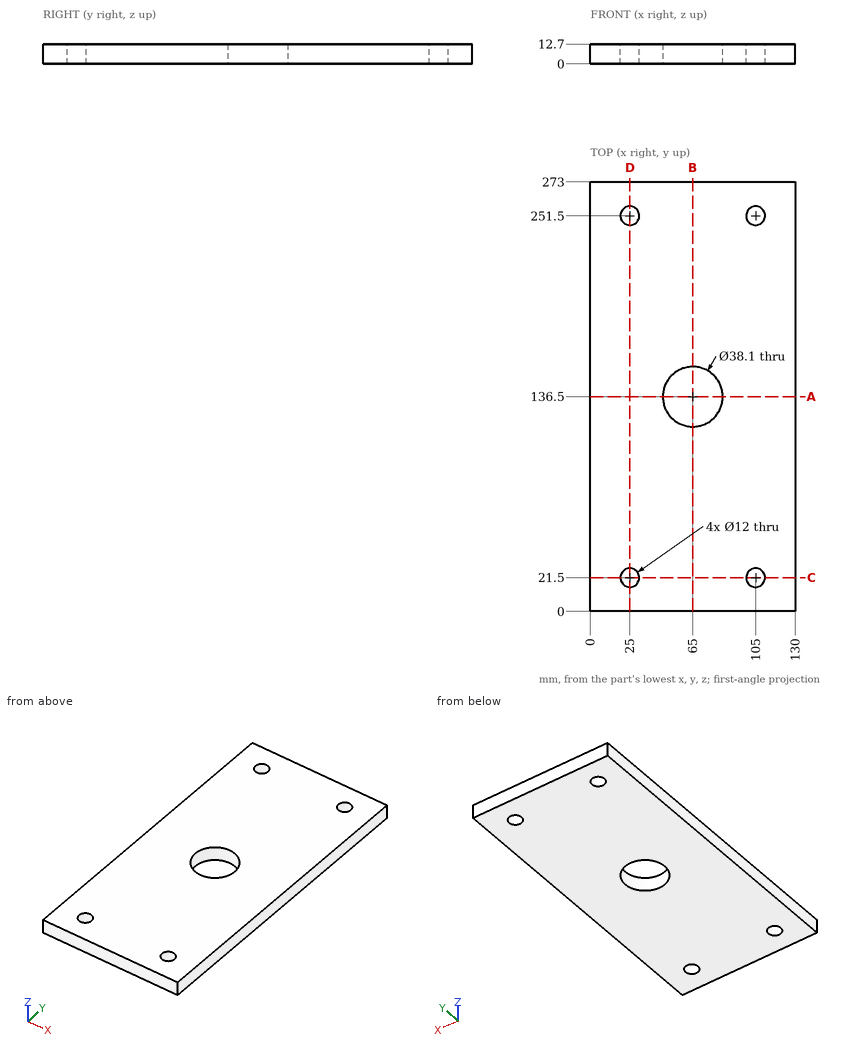
Could you check a few things on this drawing? It's one solid part, dimensions in mm from its lowest x, y, z. Coordinates: 2 decimals unless noted, no trailing zeros. Order: outer loops, then holes, each group sorted by start corner. A loop starts at its lowest first (then second) coordinate and runs counter-clockwise, first axis right, second up. Notation, with made-up numbers: (45, 2) -> (72, 2) arc R16 cw to (72, 33) -> close; hole circle Ø7 at (-18.75, -21). An arc over 180 degrees is marked (long way). Answer in a Markdown table with one row per item.
(1) I want a section at C-C on y = 21.5. List the corners of the cut face in (x, z) for me.
Answer key:
| item | result |
|---|---|
| outline | (0, 0) -> (19, 0) -> (19, 12.7) -> (0, 12.7) -> close; (31, 0) -> (99, 0) -> (99, 12.7) -> (31, 12.7) -> close; (111, 0) -> (130, 0) -> (130, 12.7) -> (111, 12.7) -> close |
(2) Please list where these lines run through material, in increasing order: probe 1 along Y at (x, z) = (105, 5.25); probe 2 along X at (y, z) = (21.5, 9.5); probe 3 along Y at (x, z) = (65, 8.25).
Answer key:
| item | result |
|---|---|
| probe 1 | 0 to 15.5, 27.5 to 245.5, 257.5 to 273 |
| probe 2 | 0 to 19, 31 to 99, 111 to 130 |
| probe 3 | 0 to 117.45, 155.55 to 273 |
(3) I want a section at B-B on x = 65. List the corners of the cut face in (y, z) for me, then the cut area to 3 significant figures.
Answer key:
| item | result |
|---|---|
| outline | (0, 0) -> (117.45, 0) -> (117.45, 12.7) -> (0, 12.7) -> close; (155.55, 0) -> (273, 0) -> (273, 12.7) -> (155.55, 12.7) -> close |
| area | 2,980 mm^2 |
(4) Will these pins go through, and if not, where does the flat tip stop? pin 1 Ø3 at (x, z) = (33, 8) entering from -Y; pin 2 Ø11 at (x, y) = (25, 251.5) entering from +Z.
Answer key:
| item | result |
|---|---|
| pin 1 | y = 0 |
| pin 2 | through |
(5) I want a section at A-A on y = 136.5. List the corners of the cut face in (x, z) for me.
Answer key:
| item | result |
|---|---|
| outline | (0, 0) -> (45.95, 0) -> (45.95, 12.7) -> (0, 12.7) -> close; (84.05, 0) -> (130, 0) -> (130, 12.7) -> (84.05, 12.7) -> close |
(6) I want a section at D-D on x = 25. List the corners of the cut face in (y, z) for me, then the cut area to 3 significant figures.
Answer key:
| item | result |
|---|---|
| outline | (0, 0) -> (15.5, 0) -> (15.5, 12.7) -> (0, 12.7) -> close; (27.5, 0) -> (245.5, 0) -> (245.5, 12.7) -> (27.5, 12.7) -> close; (257.5, 0) -> (273, 0) -> (273, 12.7) -> (257.5, 12.7) -> close |
| area | 3,160 mm^2 |
